```python
from build123d import *

# Parameters (mm, degrees)
F0_W     = 3.5306
F0_H     = 3.9528298268
F1_DEPTH = 0.79375
F2_DEPTH = 3.81
F3_W     = 3.5306
F3_H     = 3.9528298268
F4_DEPTH = 0.79375
F5_R     = 1.75
F6_DEPTH = 5.3985
F0_R     = 4.7625
F7_DEPTH = 0.79375


with BuildPart() as f1:
    # F0 (on Right) → F1 (new body)
    with BuildSketch(Plane.YZ):
        Rectangle(F0_W, F0_H)
        with BuildLine():
            Line((-1.7653, 1.9764149134), (1.7653, 1.9764149134))
            ThreePointArc((1.7653, 1.9764149134), (0.3978891493, 2.6199588212), (-1.0989290887, 2.4114010156))
            ThreePointArc((-1.0989290887, 2.4114010156), (-1.325, 2.29496732), (-1.5388699938, 2.1574010156))
            ThreePointArc((-1.5388699938, 2.1574010156), (-1.6545615218, 2.0700063214), (-1.7653, 1.9764149134))
        make_face()
        with BuildLine():
            ThreePointArc((-1.0989290887, -2.4114010156), (0.3978891493, -2.6199588212), (1.7653, -1.9764149134))
            Line((1.7653, -1.9764149134), (-1.7653, -1.9764149134))
            ThreePointArc((-1.7653, -1.9764149134), (-1.6545615218, -2.0700063214), (-1.5388699938, -2.1574010156))
            ThreePointArc((-1.5388699938, -2.1574010156), (-1.325, -2.29496732), (-1.0989290887, -2.4114010156))
        make_face()
    extrude(amount=-F1_DEPTH)

    # F0 (on Right) → F2 (join)
    with BuildSketch(Plane.YZ):
        with BuildLine():
            Line((-1.7653, 1.9764149134), (1.7653, 1.9764149134))
            ThreePointArc((1.7653, 1.9764149134), (0.3978891493, 2.6199588212), (-1.0989290887, 2.4114010156))
            ThreePointArc((-1.0989290887, 2.4114010156), (-1.325, 2.29496732), (-1.5388699938, 2.1574010156))
            ThreePointArc((-1.5388699938, 2.1574010156), (-1.6545615218, 2.0700063214), (-1.7653, 1.9764149134))
        make_face()
        with BuildLine():
            ThreePointArc((2.6377990826, -0.254), (2.6469480132, -0.1271464337), (2.65, 0))
            ThreePointArc((2.65, 0), (2.6469480132, 0.1271464337), (2.6377990826, 0.254))
            ThreePointArc((2.6377990826, 0.254), (2.3640005639, 1.1974979473), (1.7653, 1.9764149134))
            Line((1.7653, 1.9764149134), (1.7653, -1.9764149134))
            ThreePointArc((1.7653, -1.9764149134), (2.3640005639, -1.1974979473), (2.6377990826, -0.254))
        make_face()
        with BuildLine():
            Line((-1.7653, -1.9764149134), (-1.7653, 1.9764149134))
            ThreePointArc((-1.7653, 1.9764149134), (-2.65, 0), (-1.7653, -1.9764149134))
        make_face()
        Rectangle(F0_W, F0_H)
        with BuildLine():
            ThreePointArc((-1.0989290887, -2.4114010156), (0.3978891493, -2.6199588212), (1.7653, -1.9764149134))
            Line((1.7653, -1.9764149134), (-1.7653, -1.9764149134))
            ThreePointArc((-1.7653, -1.9764149134), (-1.6545615218, -2.0700063214), (-1.5388699938, -2.1574010156))
            ThreePointArc((-1.5388699938, -2.1574010156), (-1.325, -2.29496732), (-1.0989290887, -2.4114010156))
        make_face()
    extrude(amount=F2_DEPTH)

    # F3 (on face) → F4 (join)
    with BuildSketch(Plane.YZ.offset(3.81)):
        Rectangle(F3_W, F3_H)
        with BuildLine():
            ThreePointArc((1.7653, 1.9764149134), (0, 2.65), (-1.7653, 1.9764149134))
            Line((-1.7653, 1.9764149134), (1.7653, 1.9764149134))
        make_face()
        with BuildLine():
            Line((1.7653, -1.9764149134), (-1.7653, -1.9764149134))
            ThreePointArc((-1.7653, -1.9764149134), (0, -2.65), (1.7653, -1.9764149134))
        make_face()
    extrude(amount=F4_DEPTH)

    # F5 (on face) → F6 (cut, through all)
    with BuildSketch(Plane.YZ.offset(4.60375)):
        Circle(F5_R)
    extrude(amount=-F6_DEPTH, mode=Mode.SUBTRACT)

    # F0 (on Right) → F7 (join, symmetric)
    with BuildSketch(Plane.YZ):
        Circle(F0_R)
        with BuildLine():
            ThreePointArc((-1.6161623386, 3.6247752838), (1.984375, 3.4370383213), (3.9472286481, 0.41275))
            ThreePointArc((3.9472286481, 0.41275), (3.9633660101, 0.2066553478), (3.96875, 0))
            ThreePointArc((3.96875, 0), (3.9633660101, -0.2066553478), (3.9472286481, -0.41275))
            ThreePointArc((3.9472286481, -0.41275), (1.984375, -3.4370383213), (-1.6161623386, -3.6247752838))
            ThreePointArc((-1.6161623386, -3.6247752838), (-1.984375, -3.4370383213), (-2.3310663094, -3.2120252838))
            ThreePointArc((-2.3310663094, -3.2120252838), (-3.96875, 0), (-2.3310663094, 3.2120252838))
            ThreePointArc((-2.3310663094, 3.2120252838), (-1.984375, 3.4370383213), (-1.6161623386, 3.6247752838))
        make_face(mode=Mode.SUBTRACT)
        with BuildLine():
            ThreePointArc((2.6377990826, 0.254), (2.6469480132, 0.1271464337), (2.65, 0))
            ThreePointArc((2.65, 0), (2.6469480132, -0.1271464337), (2.6377990826, -0.254))
            Line((2.6377990826, -0.254), (3.1480569305, -0.41275))
            Line((3.1480569305, -0.41275), (3.9472286481, -0.41275))
            ThreePointArc((3.9472286481, -0.41275), (3.9633660101, -0.2066553478), (3.96875, 0))
            ThreePointArc((3.96875, 0), (3.9633660101, 0.2066553478), (3.9472286481, 0.41275))
            Line((3.9472286481, 0.41275), (3.1480569305, 0.41275))
            Line((3.1480569305, 0.41275), (2.6377990826, 0.254))
        make_face()
        with BuildLine():
            ThreePointArc((-1.5388699938, 2.1574010156), (-1.325, 2.29496732), (-1.0989290887, 2.4114010156))
            Line((-1.0989290887, 2.4114010156), (-1.2165764798, 2.9326722743))
            Line((-1.2165764798, 2.9326722743), (-1.6161623386, 3.6247752838))
            ThreePointArc((-1.6161623386, 3.6247752838), (-1.984375, 3.4370383213), (-2.3310663094, 3.2120252838))
            Line((-2.3310663094, 3.2120252838), (-1.9314804506, 2.5199222743))
            Line((-1.9314804506, 2.5199222743), (-1.5388699938, 2.1574010156))
        make_face()
        with BuildLine():
            Line((-1.2165764798, -2.9326722743), (-1.0989290887, -2.4114010156))
            ThreePointArc((-1.0989290887, -2.4114010156), (-1.325, -2.29496732), (-1.5388699938, -2.1574010156))
            Line((-1.5388699938, -2.1574010156), (-1.9314804506, -2.5199222743))
            Line((-1.9314804506, -2.5199222743), (-2.3310663094, -3.2120252838))
            ThreePointArc((-2.3310663094, -3.2120252838), (-1.984375, -3.4370383213), (-1.6161623386, -3.6247752838))
            Line((-1.6161623386, -3.6247752838), (-1.2165764798, -2.9326722743))
        make_face()
    extrude(amount=F7_DEPTH, both=True)


solid = f1.part
```
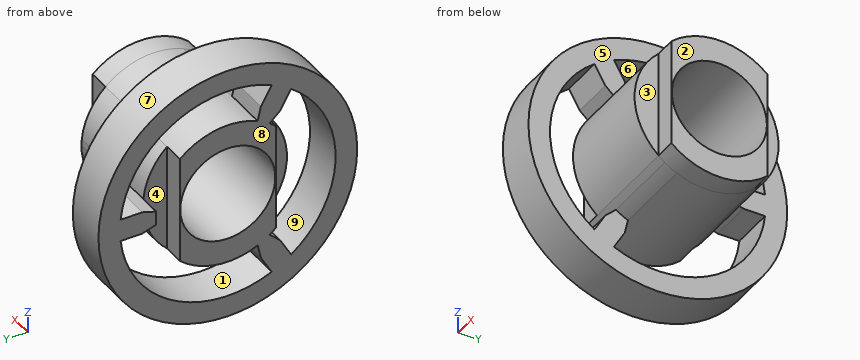
Check sheet for the modelled part. Datum: model origin and axes. Units: mm. Face numbers are marked on the shaded views. A direction names the side the tool comes from. Round coordinates to 2 decimals unless told otherwise and drop trailing zeros. Loops run counter-clockwise (first coordinate to the right, second up) from the corner with the lowest first, then second, coordinate; pieces in that order, holes last. Notation, with made-up numbers: (6, -5.75) -> (63, -5.75) arc R23 ccw to (63, 5.25) -> close; hole circle Ø3 at (88, 42). An arc over 180 degrees is marked (long way). Answer in a Markdown table with one row per item.
Q1. Go/stop test with flat-tipped pins: P1, Ø3, axis at x = 3.5, y = 2.5, coming from the +Z side; P2, Ø3, axis at x = 3.5, y = 1, coming from the +Z side; P3, Ø2, axis at x = 0.5, y = -1.5, coming from the +Z side. Record where each tip stops, or that it passes through.
Data:
| item | result |
|---|---|
| P1 | stops at z = 2.45 |
| P2 | stops at z = 2.65 |
| P3 | stops at z = 4.74 |
Q2. Sectioned sample at B-B on y = 0. Enter the section's corners in (x, z), then the cut area to 3 significant figures.
Data:
| item | result |
|---|---|
| outline | (-0.79, -4.76) -> (0.79, -4.76) -> (0.79, -3.97) -> (-0.79, -3.97) -> close; (-0.79, -2.65) -> (4.6, -2.65) -> (4.6, -1.75) -> (-0.79, -1.75) -> close; (-0.79, 1.75) -> (4.6, 1.75) -> (4.6, 2.65) -> (-0.79, 2.65) -> close; (-0.79, 3.97) -> (0.79, 3.97) -> (0.79, 4.76) -> (-0.79, 4.76) -> close |
| area | 12.2 mm^2 |
Q3. Thickness scan on L1, parallel to Z at x = 2.3, y = 0; L2, parallel to Z at x = 0.75, y = 2.25; L3, parallel to Z at x = 0.1, y = -1.5. Record the ranges inside material, lowest first.
Data:
| item | result |
|---|---|
| L1 | z = -2.65 to -1.75, 1.75 to 2.65 |
| L2 | z = -4.2 to -3.27, -1.4 to 1.4, 3.27 to 4.2 |
| L3 | z = -4.52 to -3.67, -3.42 to -0.9, 0.9 to 3.42, 3.67 to 4.52 |
Q4. Sectioned sample at D-D on z = -1.5. Enter the section's corners in (x, y).
Data:
| item | result |
|---|---|
| outline | (-0.79, -4.52) -> (0.79, -4.52) -> (0.79, -3.67) -> (-0.79, -3.67) -> close; (-0.79, -1.77) -> (0, -1.77) -> (0, -2.18) -> (3.81, -2.18) -> (3.81, -1.77) -> (4.6, -1.77) -> (4.6, -0.9) -> (-0.79, -0.9) -> close; (-0.79, 0.9) -> (4.6, 0.9) -> (4.6, 1.77) -> (3.81, 1.77) -> (3.81, 2.18) -> (0, 2.18) -> (0, 1.77) -> (-0.79, 1.77) -> close; (-0.79, 3.67) -> (0.79, 3.67) -> (0.79, 4.52) -> (-0.79, 4.52) -> close |
Q5. Set-up check for the marked faces 1, 2, 3, 4 and 5: record each of +Z, -Z, +X, -X, +Y, -Y from which the full face is reachable in a straight line by a thin tool's end or side.
Data:
| item | result |
|---|---|
| face 1 | +X, -X |
| face 2 | +Z, -Z, +X, +Y, -Y |
| face 3 | +Z, -Z, +X, -Y |
| face 4 | -X |
| face 5 | +X |
Q6. Sectioned sample at C-C on x = 0.45. Give the number of separate pieces and of enclosed holes in the cut face, then the cut area to 3 significant figures.
Data:
| item | result |
|---|---|
| separate pieces | 1 |
| enclosed holes | 4 |
| area | 37.2 mm^2 |
Q7. Release check for a two-part mould opening along Z. For the marked faces 6, 7, 8 and 9 record: released by +Z, released by -Z, zero draft, split by the parting line, or undercut.
Data:
| item | result |
|---|---|
| face 6 | undercut |
| face 7 | split by the parting line |
| face 8 | zero draft |
| face 9 | undercut |
Q8. Sectioned sample at A-A on x = 1. Enter the section's corners in (y, z).
Data:
| item | result |
|---|---|
| outline | circle Ø5.3 at (0, 0); hole circle Ø3.5 at (0, 0) |
